The listing builds one solid part. Answer for the finished solid, in the listing's coordinates (mm). Face numbers are marked on the shaded views. Coordinates: 2 decimals unless noted, no trailing zeros. Write each loop counter-clockwise with the first axis right and the second up, starting at its lowest first coordinate (ties: lowest second). Pieces come first, ordered by that corner, then holes. Notation, with made-up numbers: M 63,54 L 78,54 A13 cw 78,59 Z; hole C 52.5,64.25 d2. An arc over 180 degrees is marked long. Answer as a JSON object with one key per item and string values. Group by question number.
from build123d import *

# Parameters (mm, degrees)
BOSS_EXTRUDE1_DEPTH = 2
SKETCH9_R           = 5.15
CUT_EXTRUDE3_DEPTH  = 127.587914115
VISION_PATTERN_R    = 25
VISION_PATTERN_R_2  = 20
CUT_EXTRUDE4_DEPTH  = 127.587914115
FILLET1_R           = 10
BOSS_EXTRUDE4_DEPTH = 50
SKETCH12_W          = 60
SKETCH12_H          = 105
CUT_EXTRUDE5_DEPTH  = 1
SKETCH16_R          = 12.5
CUT_EXTRUDE9_DEPTH  = 20
SKETCH17_R          = 0.75
BOSS_EXTRUDE3_DEPTH = 0.425
FILLET2_R           = 0.4


with BuildPart() as part:
    # Sketch1 → Boss-Extrude1 (new body)
    with BuildSketch(Plane(origin=(0, 0, 0), x_dir=(1, 0, 0), z_dir=(0, 1, 0))):
        with BuildLine():
            Line((-48.839021284, -75), (48.839021284, -75))
            ThreePointArc((48.839021284, -75), (0, 89.5), (-48.839021284, -75))
        make_face()
    extrude(amount=-BOSS_EXTRUDE1_DEPTH)

    # Sketch9 → Cut-Extrude3 (cut, through all)
    with BuildSketch(Plane(origin=(0, 0, 0), x_dir=(1, 0, 0), z_dir=(0, 1, 0))):
        with Locations(Location((78.541209232, -8.501673503, 0), (0, 0, 270))):
            Circle(SKETCH9_R)
        with Locations(Location((-78.541209232, -8.501673503, 0), (0, 0, 270))):
            Circle(SKETCH9_R)
    extrude(amount=-CUT_EXTRUDE3_DEPTH, mode=Mode.SUBTRACT)

    # Vision Pattern → Cut-Extrude4 (cut, through all)
    with BuildSketch(Plane(origin=(0, 0, 0), x_dir=(1, 0, 0), z_dir=(0, 1, 0))):
        with Locations(Location((0, 0, 0), (0, 0, 270))):
            Circle(VISION_PATTERN_R)
        with Locations(Location((54.772255751, -35, 0), (0, 0, 270))):
            Circle(VISION_PATTERN_R_2)
        with Locations(Location((-54.772255751, -35, 0), (0, 0, 270))):
            Circle(VISION_PATTERN_R_2)
        with Locations(Location((35, 54.772255751, 0), (0, 0, 270))):
            Circle(VISION_PATTERN_R_2)
        with Locations(Location((-35, 54.772255751, 0), (0, 0, 270))):
            Circle(VISION_PATTERN_R_2)
    extrude(amount=-CUT_EXTRUDE4_DEPTH, mode=Mode.SUBTRACT)

    # Fillet1
    fillet1_edges = [part.edges().sort_by_distance(p)[0] for p in [
        (48.839021284, -1, 75),
        (-48.839021284, -1, 75),
    ]]
    fillet(fillet1_edges, radius=FILLET1_R)

    # Sketch18 → Boss-Extrude4 (add)
    with BuildSketch(Plane.XY.offset(5)):
        Polygon((63.11284211, -3.45), (66.88715789, -3.45), (66.05, -2), (63.95, -2), align=None)
    boss_extrude4 = extrude(amount=-BOSS_EXTRUDE4_DEPTH)

    # Mirror2: Boss-Extrude4 across plane
    add(boss_extrude4.mirror(Plane(origin=(0, 0, 0), x_dir=(0, 0, 1), z_dir=(1, 0, 0))))

    # Sketch12 → Cut-Extrude5 (cut)
    with BuildSketch(Plane.XZ.offset(2)):
        with Locations((0, 22.5)):
            Rectangle(SKETCH12_W, SKETCH12_H)
    extrude(amount=-CUT_EXTRUDE5_DEPTH, mode=Mode.SUBTRACT)

    # Sketch16 → Cut-Extrude9 (cut)
    with BuildSketch(Plane(origin=(0, 0, 0), x_dir=(1, 0, 0), z_dir=(0, 1, 0))):
        with Locations((0, -75)):
            Circle(SKETCH16_R)
    extrude(amount=-CUT_EXTRUDE9_DEPTH, mode=Mode.SUBTRACT)

    # Sketch17 → Boss-Extrude3 (add)
    with BuildSketch(Plane.XZ.offset(1)):
        with Locations(Location((-20, 72.05, 0), (0, 0, 270))):
            Circle(SKETCH17_R)
    boss_extrude3 = extrude(amount=BOSS_EXTRUDE3_DEPTH)

    # Mirror1: Boss-Extrude3 across plane
    add(boss_extrude3.mirror(Plane(origin=(0, 0, 0), x_dir=(0, 0, 1), z_dir=(1, 0, 0))))

    # Fillet2
    fillet2_edges = [part.edges().sort_by_distance(p)[0] for p in [
        (-20, -1.425, 72.8),
        (20, -1.425, 72.8),
    ]]
    fillet(fillet2_edges, radius=FILLET2_R)


solid = part.part
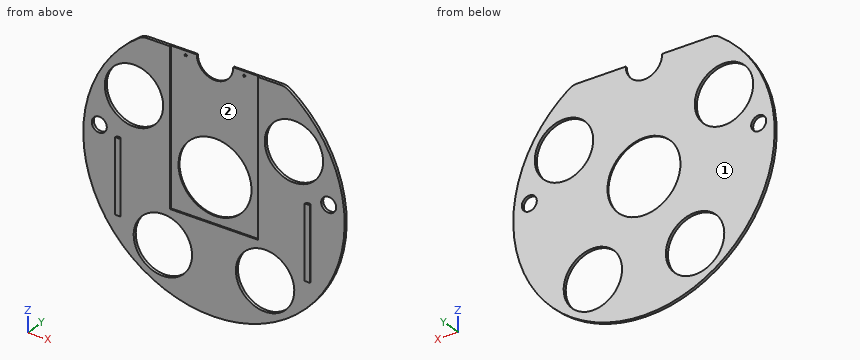
Item 1: A cutting plane is placed at C-C, the plane y = -2.9. Write down the section's boundary in (x, z), and give its area (3 significant figures).
Item 2: Flat-ended cylindrical pins translate along their axes: pin 1 Ø10 at (x, z) = (-15.5, 19) entering from -Y; pin 2 Ø1.6 at (x, y) = (65.5, -2.5) entering from -Z; pin 3 Ø1 at (x, y) = (64.5, -1.5) entering from +Z; pin 4 Ø24 at (x, z) = (-54.77, 35) entering from +Y. Find the tip coordinate at first contact, or state that the pin passes through.
Item 3: For a pull along X with two mould halves and no side action, classify the marked faces 1 and 2 as +X half, -X half, draft (parallel to the pull), parting line (faces both ways), or undercut.
Item 4: A cutting plane is placed at B-B, the plane z = 38.5. Write down the section's boundary in (x, y), and give its area (3 significant figures).
Item 5: A cutting plane is placed at D-D, the plane x = -42.5. Write down the section's boundary in (y, z), and give its area (3 significant figures).
Item 6: Consider L1, parallel to X at y = -0.9, z = 22.5; L2, parallel to X at y = -1.55, z = 26; L3, parallel to Z at x = 47.5, y = -0.85. Determine where each line is inside the solid, lowest interval first. Write a range as from..to.
Item 7: A cutting plane is placed at A-A, the plane x = 0. Write down the section's boundary in (y, z).
Answer:
{
 "1": {"outline": "M -66.57,-45 L -63.43,-45 L -63.43,5 L -66.57,5 Z; M 63.43,-45 L 66.57,-45 L 66.57,5 L 63.43,5 Z", "area": "314 mm2"},
 "2": {"pin 1": "y = -1", "pin 2": "z = -61.66", "pin 3": "z = 62.56", "pin 4": "through"},
 "3": {"face 1": "draft", "face 2": "undercut"},
 "4": {"outline": "M -80.8,-2 L -74.46,-2 L -74.46,0 L -80.8,0 Z; M -35.08,-2 L -30,-2 L -30,-1 L 30,-1 L 30,-2 L 35.08,-2 L 35.08,0 L -35.08,0 Z; M 74.46,-2 L 80.8,-2 L 80.8,0 L 74.46,0 Z", "area": "106 mm2"},
 "5": {"outline": "M -2,-78.77 L 0,-78.77 L 0,-73.31 L -2,-73.31 Z; M -2,-36.23 L 0,-36.23 L 0,19.21 L -2,19.21 Z; M -2,50.79 L 0,50.79 L 0,75 L -2,75 Z", "area": "170 mm2"},
 "6": {"L1": "-86.63..-70.38, -39.16..-10.9, 10.9..39.16, 70.38..86.63", "L2": "-85.64..-72.63, -36.91..-30, 30..36.91, 72.63..85.64", "L3": "-75.86..-70.38, -39.16..16.37, 53.63..74.85"},
 "7": {"outline": "M -2,-89.5 L 0,-89.5 L 0,-25 L -1,-25 L -1,-30 L -2,-30 Z; M -1,25 L 0,25 L 0,62.5 L -1,62.5 Z"}
}
